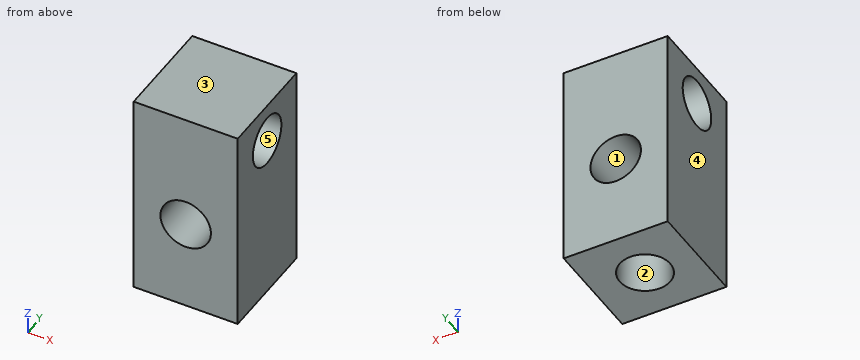
```python
from build123d import *

# Parameters (mm, degrees)
SKETCH1_W                       = 10
SKETCH1_H                       = 9.970930233
BOSS_EXTRUDE1_DEPTH             = 20
F_11_0_191_DIAMETER_HOLE6_D     = 4.8514
F_11_0_191_DIAMETER_HOLE6_DEPTH = 4
F_11_0_191_DIAMETER_HOLE6_TIP   = 1.457507604
F_11_0_191_DIAMETER_HOLE7_D     = 4.8514
F_11_0_191_DIAMETER_HOLE8_D     = 4.8514


with BuildPart() as part:
    # Sketch1 → Boss-Extrude1 (new body)
    with BuildSketch(Plane.XY):
        with Locations((-5, 4.985465117)):
            Rectangle(SKETCH1_W, SKETCH1_H)
    extrude(amount=BOSS_EXTRUDE1_DEPTH)

    # #11 (0.191) Diameter Hole6
    with Locations(Plane(origin=(0, 0, 0), x_dir=(-1, 0, 0), z_dir=(0, 0, -1))):
        with Locations((5, 4.985465116)):
            Hole(F_11_0_191_DIAMETER_HOLE6_D / 2, depth=F_11_0_191_DIAMETER_HOLE6_DEPTH)
            with Locations((0, 0, -(F_11_0_191_DIAMETER_HOLE6_DEPTH + F_11_0_191_DIAMETER_HOLE6_TIP / 2))):  # 118° drill point
                Cone(0, F_11_0_191_DIAMETER_HOLE6_D / 2, F_11_0_191_DIAMETER_HOLE6_TIP, mode=Mode.SUBTRACT)

    # #11 (0.191) Diameter Hole7 (through all)
    with Locations(Plane(origin=(0, 9.970930233, 0), x_dir=(1, 0, 0), z_dir=(0, 1, 0))):
        with Locations((-5, -8.75)):
            Hole(F_11_0_191_DIAMETER_HOLE7_D / 2)

    # #11 (0.191) Diameter Hole8 (through all)
    with Locations(Plane.ZY.offset(10)):
        with Locations((16.25, 5)):
            Hole(F_11_0_191_DIAMETER_HOLE8_D / 2)


solid = part.part
```
Source: CAD feature listing. Evaluate the final solid. Frame: model axes, mm. Face numbers are marked on the shaded views. A direction names the side the tool comes from. Round coordinates to 2 decimals unless told otherwise and drop trailing zeros. Loops run counter-clockwise (first coordinate to the right, second up) from the corner with the lowest first, then second, coordinate; pieces in that order, holes last.
(1) Section query C-C (y = 8). Output: boundary loops of the cut face in (x, z).
From the geometry:
outline: (-10, 0) - (0, 0) - (0, 20) - (-10, 20) - close; hole circle Ø4.85 at (-5, 8.75)
(2) Section query A-A (z = 8.75). Output: boundary loops of the cut face in (x, y), and give its area (3 significant figures).
From the geometry:
outline: (-10, 0) - (-7.43, 0) - (-7.43, 9.97) - (-10, 9.97) - close; (-2.57, 0) - (0, 0) - (0, 9.97) - (-2.57, 9.97) - close
area: 51.3 mm2
(3) Section query B-B (x = -7.75). Output: boundary loops of the cut face in (y, z).
From the geometry:
outline: (0, 0) - (9.97, 0) - (9.97, 20) - (0, 20) - close; hole circle Ø4.85 at (5, 16.25)
(4) Pull-direction query (Z, two-part tool) for the marked faces 3, 4 and 5; classes: +Z half, -Z half, draft (parallel to the pull), parting line (faces both ways), or undercut.
From the geometry:
face 3: +Z half
face 4: draft
face 5: undercut
(5) Access query for the marked faces 1 and 2. Directions: +Z, -Z, +X, -X, +Y, -Y. A direction counts if a zero-diameter tool reaches every point of the face in a straight line with its end or side. Return the directions, or none.
From the geometry:
face 1: +Y, -Y
face 2: -Z
(6) Material intervals for probe 1 along Z at (x, y) = (-3, 6.5); probe 2 along Z at (x, y) = (-4.25, 6.25); probe 3 along X at (y, z) = (4, 8.75), sorted ascending.
From the geometry:
probe 1: z = 0 to 7.38, 10.12 to 14.34, 18.16 to 20
probe 2: z = 4.57 to 6.44, 11.06 to 14.17, 18.33 to 20
probe 3: x = -10 to -7.43, -2.57 to 0
(7) Section query D-D (x = -3.75). Give the number of separate pieces and of enclosed holes in the cut face, and give its area (3 significant figures).
From the geometry:
separate pieces: 2
enclosed holes: 1
area: 121 mm2
